Verification items for this drawing (mm, ordinates from the low corner). A direction names the side the tool comes from. Round coordinates to 2 decimals unless told otherwise and drop trailing zeros. Loops run counter-clockwise (first coordinate to the right, second up) from the corner with the lowest first, then second, coordinate; pieces in that order, holes last. Notation, with made-up numbers: (38, -2) - (86, -2) arc R18 cw to (86, 3) - close; hole circle Ø7 at (-24, 86). An arc over 180 degrees is marked (long way). Answer in a Markdown table with one row per item. Add a question column.
(1) Mould release check, pull along Y, two halves, no side actions. Record for the marked faces 1, 2 and 3: +Y half, -Y half, draft (parallel to the pull), parting line (faces both ways), or undercut.
(2) Gauge pin test, flat ends, axial feed: pin 1 (4 mm diameter, centred on x = 16.5, z = 10, fed in from +Y); pin 2 (1.5 mm diameter, centred on x = 20.5, y = 2, fed in from +Z); pin 3 (1.5 mm diameter, centred on x = 11.5, y = 7, fed in from -Z). Record the tip position at first contact, or that the pin passes through.
(3) Thickness scan on line 1 along X through (y, z) = (2.25, 6.75); line 2 along Y through (x, z) = (3.25, 6); line 3 along X through (y, z) = (2, 9.75). Record the ranges inside material, lowest first.
(4) Cross-section at A-A on z = 6. Enter the section's corners in (x, y).
(5) Access from +Z, -Z, +X, -X, +Y, -Y to the whole of each face (thin tool, end or side, straight path). Record for the marked faces 4 and 5.
(6) Cross-section at D-D on x = 18.75. Enter the section's corners in (y, z), then the cut area to 3 significant figures.
(7) Cross-section at B-B on y = 5. Enter the section's corners in (x, z), then the cut area to 4 significant figures.
(8) Cross-section at C-C on x = 6. Enter the section's corners in (y, z).
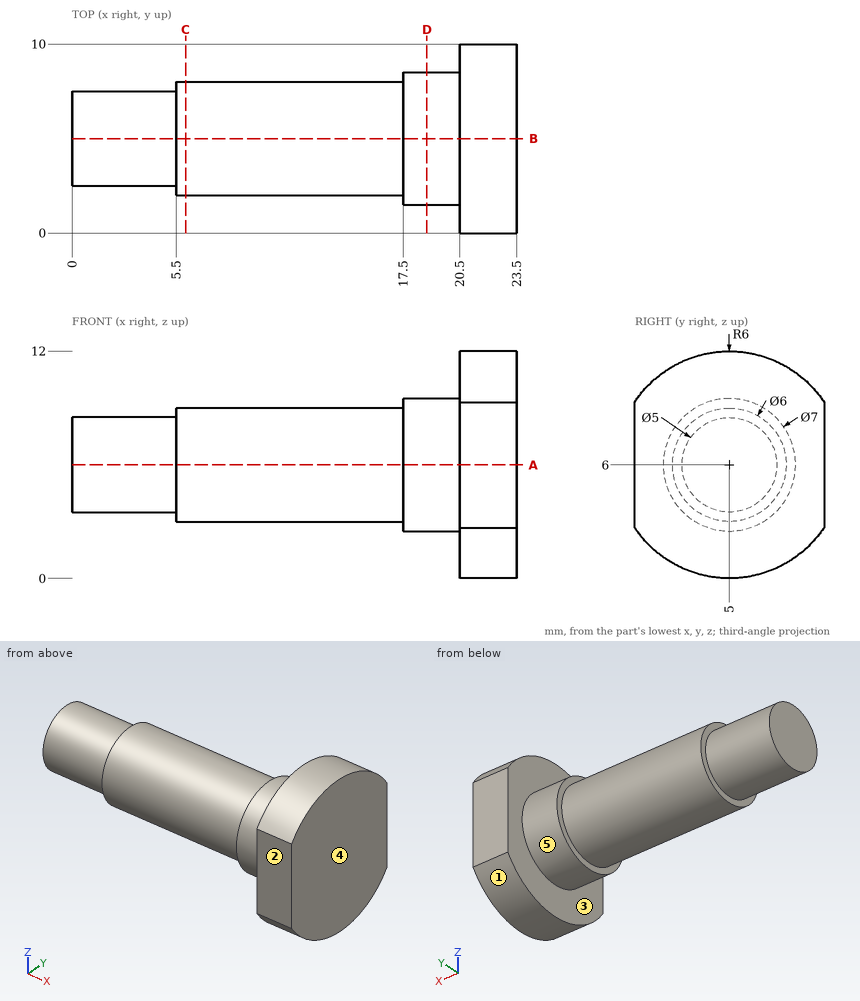
Answers:
| question | item | result |
|---|---|---|
| 1 | face 1 | parting line |
| 1 | face 2 | -Y half |
| 1 | face 3 | draft |
| 2 | pin 1 | stops at y = 7.67 |
| 2 | pin 2 | stops at z = 11.56 |
| 2 | pin 3 | stops at z = 3.27 |
| 3 | line 1 | x = 5.5 to 23.5 |
| 3 | line 2 | y = 2.5 to 7.5 |
| 3 | line 3 | x = 20.5 to 23.5 |
| 4 | outline | (0, 2.5) - (5.5, 2.5) - (5.5, 2) - (17.5, 2) - (17.5, 1.5) - (20.5, 1.5) - (20.5, 0) - (23.5, 0) - (23.5, 10) - (20.5, 10) - (20.5, 8.5) - (17.5, 8.5) - (17.5, 8) - (5.5, 8) - (5.5, 7.5) - (0, 7.5) - close |
| 5 | face 4 | +Z, -Z, +X, +Y, -Y |
| 5 | face 5 | -X |
| 6 | outline | circle Ø7 at (5, 6) |
| 6 | area | 38.5 mm^2 |
| 7 | outline | (0, 3.5) - (5.5, 3.5) - (5.5, 3) - (17.5, 3) - (17.5, 2.5) - (20.5, 2.5) - (20.5, 0) - (23.5, 0) - (23.5, 12) - (20.5, 12) - (20.5, 9.5) - (17.5, 9.5) - (17.5, 9) - (5.5, 9) - (5.5, 8.5) - (0, 8.5) - close |
| 7 | area | 156.5 mm^2 |
| 8 | outline | circle Ø6 at (5, 6) |
